Source: CAD feature listing. Evaluate the final solid. Frame: model axes, mm. A direction names the side the tool comes from. Coordinates: 2 decimals unless noted, no trailing zeros. Write each loop counter-clockwise with the first axis right and the second up, starting at its lowest first coordinate (ties: lowest second). Pieces come first, ordered by that corner, then holes. Notation, with made-up numbers: (79.25, 48) - (131.25, 48) arc R3 ccw to (131.25, 52) - close; hole circle Ø3 at (-5, 27.5). An arc over 180 degrees is marked (long way). One line per question, with ' | ' between items.
from build123d import *

# Parameters (mm, degrees)
SKETCH1_R           = 11.5062
BOSS_EXTRUDE2_DEPTH = 4.7625
BOSS_EXTRUDE3_DEPTH = 3.175
FILLET1_R           = 3.175
CHAMFER1_SIZE       = 0.889


with BuildPart() as part:
    # Sketch1 → Boss-Extrude2 (new, symmetric)
    with BuildSketch(Plane.XY):
        with BuildLine():
            ThreePointArc((14.622568956, -1.310767167), (-0.601565421, 14.668870184), (-14.466139546, -2.503685297))
            ThreePointArc((-14.466139546, -2.503685297), (0.601565421, -14.668870184), (14.622568956, -1.310767167))
        make_face()
        with Locations(Location((0, 0, 0), (0, 0, 180))):
            Circle(SKETCH1_R, mode=Mode.SUBTRACT)
    extrude(amount=BOSS_EXTRUDE2_DEPTH, both=True)

    # Sketch1_4 → Boss-Extrude3 (add, symmetric)
    with BuildSketch(Plane.XY):
        with BuildLine():
            ThreePointArc((-14.466139546, -2.503685297), (-14.311462857, -6.781419913), (-15.305325324, -10.94497317))
            Line((-15.305325324, -10.94497317), (-25.200549915, -36.491056527))
            Line((-25.200549915, -36.491056527), (-8.944132177, -42.787947613))
            ThreePointArc((-8.944132177, -42.787947613), (-6.514327997, -42.754109018), (-4.820124483, -41.012050504))
            Line((-4.820124483, -41.012050504), (-1.389891456, -32.156362789))
            ThreePointArc((-1.389891456, -32.156362789), (1.241500044, -30.27335404), (4.018239298, -31.93457717))
            Line((4.018239298, -31.93457717), (11.459775477, -47.279913889))
            ThreePointArc((11.459775477, -47.279913889), (13.276123878, -48.894216183), (15.701960247, -48.75134801))
            Line((15.701960247, -48.75134801), (31.414412198, -41.131783721))
            Line((31.414412198, -41.131783721), (16.150123108, -9.654995833))
            ThreePointArc((16.150123108, -9.654995833), (14.818679492, -5.586802595), (14.622568956, -1.310767167))
            ThreePointArc((14.622568956, -1.310767167), (0.601565421, -14.668870184), (-14.466139546, -2.503685297))
        make_face()
        with BuildLine():
            ThreePointArc((-6.67017355, -32.602949236), (-13.858222202, -35.777186892), (-17.032459858, -28.58913824))
            Line((-17.032459858, -28.58913824), (-15.353855363, -24.25555592))
            ThreePointArc((-15.353855363, -24.25555592), (-8.165806711, -21.081318264), (-4.991569055, -28.269366916))
            Line((-4.991569055, -28.269366916), (-6.67017355, -32.602949236))
        make_face(mode=Mode.SUBTRACT)
        with BuildLine():
            ThreePointArc((22.626728223, -33.925216011), (20.051718512, -41.34903936), (12.627895164, -38.774029649))
            Line((12.627895164, -38.774029649), (10.600086587, -34.59244608))
            ThreePointArc((10.600086587, -34.59244608), (13.175096297, -27.168622731), (20.598919646, -29.743632442))
            Line((20.598919646, -29.743632442), (22.626728223, -33.925216011))
        make_face(mode=Mode.SUBTRACT)
    extrude(amount=BOSS_EXTRUDE3_DEPTH, both=True)

    # Fillet1
    fillet1_edges = [part.edges().sort_by_distance(p)[0] for p in [
        (31.414412198, -41.131783721, 0),
        (-25.200549915, -36.491056527, 0),
    ]]
    fillet(fillet1_edges, radius=FILLET1_R)

    # Chamfer1
    chamfer1_edges = [part.edges().sort_by_distance(p)[0] for p in [
        (11.5062, 0, -4.7625),
        (11.5062, 0, 4.7625),
    ]]
    chamfer(chamfer1_edges, length=CHAMFER1_SIZE)


solid = part.part
Item 1: Access query for faces 1 (the face through (-16.205, -26.453, 0.044)), 2 (the face through (-3.13, -36.65, 0.04)), 3 (the face through (22.04, -45.68, 0.04)). Directions: +Z, -Z, +X, -X, +Y, -Y. A direction counts if a zero-diameter tool reaches every point of the face in a straight line with its end or side. Return the directions, or none.
Check sheet entries:
face 1: +Z, -Z | face 2: +Z, -Z, -Y | face 3: +Z, -Z, +X, -Y
Item 2: Cut plane D-D on y = 0. Return loops of the section in (x, z), and give its area (3 significant figures).
Check sheet entries:
outline: (-14.68, -4.76) - (-12.4, -4.76) - (-11.51, -3.87) - (-11.51, 3.87) - (-12.4, 4.76) - (-14.68, 4.76) - close; (11.51, -3.87) - (12.4, -4.76) - (14.68, -4.76) - (14.68, 4.76) - (12.4, 4.76) - (11.51, 3.87) - close | area: 58.9 mm²
Item 3: Mould query, pull axis X, two halves, no side actions, for faces 4 (the face through (-15.685, -40.177, 0.044)), 5 (the face through (-10, -8, -4.762)), 6 (the face through (-13.74, -35.82, 0.04)). Classes: pulls with the +X half, pulls with the -X half, needs draft (parallel to the pull), parting line crosses it, or undercut.
Check sheet entries:
face 4: pulls with the -X half | face 5: needs draft | face 6: undercut
Item 4: Ray query, line 1 along Y through (x, z) = (-8.5, -0.75); line 2 along X through (y, z) = (3, 2); line 3 along Y through (x, z) = (0, 2.5). Return the intervals inside material, ascending. Write a range as [from, to].
Check sheet entries:
line 1: [-42.93, -35.03], [-20.96, -7.76], [7.76, 11.97] | line 2: [-14.37, -11.11], [11.11, 14.37] | line 3: [-30.6, -11.51], [11.51, 14.68]
Item 5: Cut plane A-A on z = 1.5. State how many separate pieces and enclosed holes the cut face has, and give its area (3 significant figures).
Check sheet entries:
separate pieces: 1 | enclosed holes: 3 | area: 1,300 mm²
Item 6: Pin query (flat end, axial travel): pin 1 Ø6 at (x, y) = (-8, -16) entering from +Z (3 decimals); pin 2 Ø4 at (x, z) = (23.5, -3.5) entering from +Y; pin 3 Ø1.5 at (x, z) = (6, 1) entering from -Y. Return the tip coordinate at first contact, or that it passes through.
Check sheet entries:
pin 1: z = 3.175 | pin 2: y = -20.74 | pin 3: y = -37.57
Item 7: Cut plane C-C on x = 18. Return loops of the section in (y, z) (3 decimals), and give its area (3 significant figures).
Check sheet entries:
outline: (-47.637, -3.175) - (-41.893, -3.175) - (-41.893, 3.175) - (-47.637, 3.175) - close; (-27.157, -3.175) - (-13.47, -3.175) - (-13.47, 3.175) - (-27.157, 3.175) - close | area: 123 mm²
Item 8: Cut plane B-B on y = -21.5. Return loops of the section in (x, z) (3 decimals), and give its area (3 significant figures).
Check sheet entries:
outline: (-19.394, -3.175) - (-13.035, -3.175) - (-13.035, 3.175) - (-19.394, 3.175) - close; (-7.311, -3.175) - (21.894, -3.175) - (21.894, 3.175) - (-7.311, 3.175) - close | area: 226 mm²
